Part print with two shaded views. Sizes in mm from the minimum x, y, z corner. Coordinates: 2 decimals unless noted, no trailing zeros. Order: outer loops, then holes, each group sorted by start corner. A loop starts at its lowest first (then second) coordinate and runs counter-clockwise, first axis right, second up. Notation, with made-up numbers: M 30.5,-4.5 L 62.5,-4.5 A9 cw 62.5,3.5 Z; hole C -40,53 d7. An arc over 180 degrees is marked long. Answer in a Markdown table with one row per item. Add a question column.
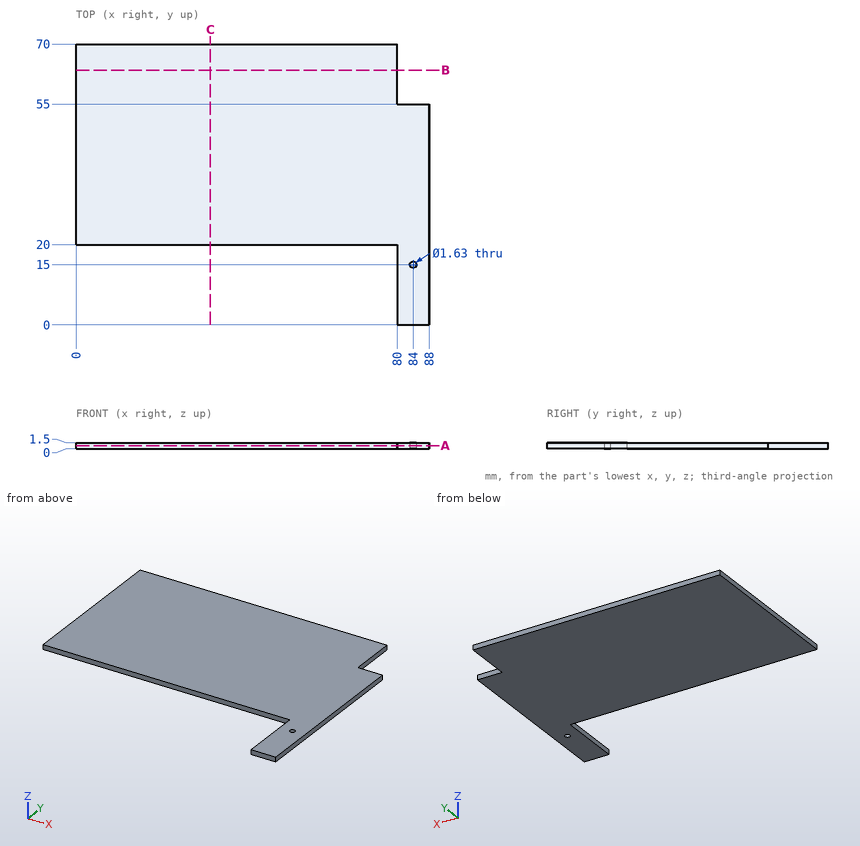
(1) Slice it at B-B (y = 63.5). List the corners of the cut face in (x, z).
(2) Slice it at C-C (x = 33.5). List the corners of the cut face in (y, z).
(3) Slice it at A-A (z = 0.8). List the corners of the cut face in (x, y) (3 decimals).
(4) Drop a flat-ended pin along its axis: P1, Ø0.8, axis at y = 61.5, z = 1, coming from the +X side. Give the stop position or say it passes through.
(5) Wall check: line 1 (X direction, y = 15, z = 0.95) (3 decimals); line 2 (Y direction, x = 84, z = 0.95) (3 decimals); line 3 (Y direction, x = 46, z = 0.75). Give the ranges that are in metal, low to high.
Computed:
| question | item | result |
|---|---|---|
| 1 | outline | M 0,0 L 80,0 L 80,1.5 L 0,1.5 Z |
| 2 | outline | M 20,0 L 70,0 L 70,1.5 L 20,1.5 Z |
| 3 | outline | M 0,20 L 80,20 L 80,0 L 88,0 L 88,55 L 80,55 L 80,70 L 0,70 Z; hole C 84,15 d1.63 |
| 4 | P1 | stops at x = 80 |
| 5 | line 1 | x = 80 to 83.185, 84.815 to 88 |
| 5 | line 2 | y = 0 to 14.185, 15.815 to 55 |
| 5 | line 3 | y = 20 to 70 |
